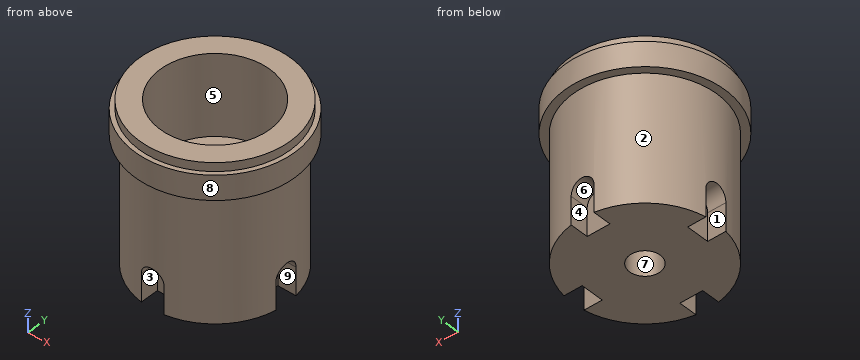
```python
from build123d import *

# Parameters (mm, degrees)
F0_R      = 15.8
F1_DEPTH  = 27.7
F2_R      = 17.5
F2_R_2    = 15.8
F3_DEPTH  = 5.4
F4_R      = 16.55
F5_DEPTH  = 1.9
F7_DEPTH  = 6.1
F8_DEPTH  = 6.1
F9_R      = 2.5
F10_DEPTH = 25
F11_DEPTH = 6.1
F12_R     = 2.5
F13_DEPTH = 25
F15_DEPTH = 25
F16_R     = 2.5
F17_DEPTH = 25
F18_R     = 12
F19_DEPTH = 17.7
F20_R     = 3.35
F21_DEPTH = 33.4


with BuildPart() as f1:
    # F0 (on Top) → F1 (new body)
    with BuildSketch(Plane.XY):
        Circle(F0_R)
    extrude(amount=F1_DEPTH)

    # F2 (on face) → F3 (join)
    with BuildSketch(Plane.XY.offset(27.7)):
        Circle(F2_R)
        Circle(F2_R_2, mode=Mode.SUBTRACT)
        Circle(F2_R_2)
    extrude(amount=F3_DEPTH)

    # F4 (on face) → F5 (join)
    with BuildSketch(Plane.XY.offset(33.1)):
        Circle(F4_R)
    extrude(amount=F5_DEPTH)

    # F6 (on face) → F7 (join)
    with BuildSketch(Plane(origin=(0, 0, 0), x_dir=(1, 0, 0), z_dir=(0, 0, -1))):
        with BuildLine():
            Line((15.6009615088, 2.5), (11.6, 2.5))
            Line((11.6, 2.5), (11.6, -2.5))
            Line((11.6, -2.5), (15.6009615088, -2.5))
            ThreePointArc((15.6009615088, -2.5), (15.7501617744, -1.2539553741), (15.8, 0))
            ThreePointArc((15.8, 0), (15.7501617744, 1.2539553741), (15.6009615088, 2.5))
        make_face()
    extrude(amount=-F7_DEPTH)

    # F6 (on face) → F8 (cut)
    with BuildSketch(Plane(origin=(0, 0, 0), x_dir=(1, 0, 0), z_dir=(0, 0, -1))):
        with BuildLine():
            Line((-2.5, 15.6009615088), (-2.5, 11.6))
            Line((-2.5, 11.6), (2.5, 11.6))
            Line((2.5, 11.6), (2.5, 15.6009615088))
            ThreePointArc((2.5, 15.6009615088), (0, 15.8), (-2.5, 15.6009615088))
        make_face()
    extrude(amount=-F8_DEPTH, mode=Mode.SUBTRACT)

    # F9 (on face) → F10 (cut)
    with BuildSketch(Plane.XZ.offset(11.6)):
        with BuildLine():
            Line((2.5, 0), (2.5, 6.1))
            ThreePointArc((2.5, 6.1), (0, 3.6), (-2.5, 6.1))
            Line((-2.5, 6.1), (-2.5, 0))
            Line((-2.5, 0), (2.5, 0))
        make_face()
        with Locations((0, 6.1)):
            Circle(F9_R)
    extrude(amount=F10_DEPTH, mode=Mode.SUBTRACT)

    # F6 (on face) → F11 (cut)
    with BuildSketch(Plane(origin=(0, 0, 0), x_dir=(1, 0, 0), z_dir=(0, 0, -1))):
        with BuildLine():
            Line((-11.6, -2.5), (-11.6, 2.5))
            Line((-11.6, 2.5), (-15.6009615088, 2.5))
            ThreePointArc((-15.6009615088, 2.5), (-15.8, 0), (-15.6009615088, -2.5))
            Line((-15.6009615088, -2.5), (-11.6, -2.5))
        make_face()
        with BuildLine():
            Line((2.5, -11.6), (-2.5, -11.6))
            Line((-2.5, -11.6), (-2.5, -15.6009615088))
            ThreePointArc((-2.5, -15.6009615088), (0, -15.8), (2.5, -15.6009615088))
            Line((2.5, -15.6009615088), (2.5, -11.6))
        make_face()
        with BuildLine():
            Line((15.6009615088, 2.5), (11.6, 2.5))
            Line((11.6, 2.5), (11.6, -2.5))
            Line((11.6, -2.5), (15.6009615088, -2.5))
            ThreePointArc((15.6009615088, -2.5), (15.7501617744, -1.2539553741), (15.8, 0))
            ThreePointArc((15.8, 0), (15.7501617744, 1.2539553741), (15.6009615088, 2.5))
        make_face()
    extrude(amount=-F11_DEPTH, mode=Mode.SUBTRACT)

    # F12 (on face) → F13 (cut)
    with BuildSketch(Plane(origin=(-11.6, 0, 0), x_dir=(0, -1, 0), z_dir=(-1, 0, 0))):
        with Locations((0, 6.1)):
            Circle(F12_R)
    extrude(amount=F13_DEPTH, mode=Mode.SUBTRACT)

    # F14 (on face) → F15 (cut)
    with BuildSketch(Plane(origin=(0, 11.6, 0), x_dir=(-1, 0, 0), z_dir=(0, 1, 0))):
        with BuildLine():
            Line((-2.5, 6.1), (2.5, 6.1))
            ThreePointArc((2.5, 6.1), (0, 8.6), (-2.5, 6.1))
        make_face()
    extrude(amount=F15_DEPTH, mode=Mode.SUBTRACT)

    # F16 (on face) → F17 (cut)
    with BuildSketch(Plane.YZ.offset(11.6)):
        with Locations((0, 6.1)):
            Circle(F16_R)
    extrude(amount=F17_DEPTH, mode=Mode.SUBTRACT)

    # F18 (on face) → F19 (cut)
    with BuildSketch(Plane.XY.offset(35)):
        Circle(F18_R)
    extrude(amount=-F19_DEPTH, mode=Mode.SUBTRACT)

    # F20 (on face) → F21 (cut)
    with BuildSketch(Plane.XY.offset(17.3)):
        Circle(F20_R)
    extrude(amount=-F21_DEPTH, mode=Mode.SUBTRACT)


solid = f1.part
```
Geometry check sheet. Reference: the model listing, model coordinates, mm. Face numbers are marked on the shaded views. A direction names the side the tool comes from. Coordinates: 2 decimals unless noted, no trailing zeros. Loops run counter-clockwise (first coordinate to the right, second up) from the corner with the lowest first, then second, coordinate; pieces in that order, holes last.
Item 1: Release check for a two-part mould opening along X. For the marked faces 6, 7, 8 and 9 record: released by +X, released by -X, zero draft, split by the parting line, or undercut.
Item 2: Thickness scan on line 1 (Y direction, x = 0, z = 11); line 2 (Y direction, x = 0, z = 4.75); line 3 (Z direction, x = 4.5, y = 5.5). Record the ranges inside material, lowest first.
Item 3: Sectioned sample at A-A, the plane x = 0. Record the boundary of the cut face in (y, z).
Item 4: Access from +Z, -Z, +X, -X, +Y, -Y to the whole of each face (thin tool, end or side, straight path). Record for the marked faces 1, 2, 3, 4 and 5.
Item 5: Sectioned sample at C-C, the plane z = 16.5. Record the boundary of the cut face in (x, y).
Item 6: Go/stop test with flat-tipped pins: pin 1 Ø4.5 at (x, z) = (14, 3) entering from -Y; pin 2 Ø2 at (x, z) = (-6.5, 7.5) entering from -Y; pin 3 Ø1.2 at (x, z) = (-14, 3.5) entering from -Y; pin 4 Ø6 at (x, y) = (0, 0) entering from +Z. Record where each tip stops, or that it passes through.
Item 7: Sectioned sample at D-D, the plane x = -10.5. Record the boundary of the cut face in (y, z), then the cut area to 3 significant figures.
Check result:
1. face 6: undercut
1. face 7: undercut
1. face 8: split by the parting line
1. face 9: zero draft
2. line 1: y = -15.8 to -3.35, 3.35 to 15.8
2. line 2: y = -11.6 to -3.35, 3.35 to 11.6
2. line 3: z = 0 to 17.3
3. outline: (-17.5, 27.7) - (-15.8, 27.7) - (-15.8, 8.6) - (-11.6, 8.6) - (-11.6, 0) - (-3.35, 0) - (-3.35, 17.3) - (-12, 17.3) - (-12, 35) - (-16.55, 35) - (-16.55, 33.1) - (-17.5, 33.1) - close; (3.35, 0) - (11.6, 0) - (11.6, 8.6) - (15.8, 8.6) - (15.8, 27.7) - (17.5, 27.7) - (17.5, 33.1) - (16.55, 33.1) - (16.55, 35) - (12, 35) - (12, 17.3) - (3.35, 17.3) - close
4. face 1: -Z, -X
4. face 2: -Z
4. face 3: -Z, -Y
4. face 4: -Z, +Y
4. face 5: +Z
5. outline: circle Ø31.6 at (0, 0); hole circle Ø6.7 at (0, 0)
6. pin 1: stops at y = -10.56
6. pin 2: stops at y = -14.81
6. pin 3: stops at y = -8.37
6. pin 4: passes through
7. outline: (-14, 27.7) - (-11.81, 27.7) - (-11.81, 0) - (11.81, 0) - (11.81, 27.7) - (14, 27.7) - (14, 33.1) - (12.79, 33.1) - (12.79, 35) - (5.81, 35) - (5.81, 17.3) - (-5.81, 17.3) - (-5.81, 35) - (-12.79, 35) - (-12.79, 33.1) - (-14, 33.1) - close
7. area: 648 mm2
